The model under review builds one solid part; all positions refer to its coordinate system, in mm. A direction names the side the tool comes from. Round coordinates to 2 decimals unless told otherwise and drop trailing zeros. Order: outer loops, then holes, each group sorted by start corner. A loop starts at its lowest first (then second) coordinate and runs counter-clockwise, first axis right, second up. Notation, with made-up numbers: (64, -22.75) -> (70, -22.75) arc R12 cw to (70, -11.75) -> close; hole circle Ø5 at (32.5, 49). An arc over 180 degrees is marked (long way). Return JSON: item names as keys, results as strings. Group by question number.
from build123d import *

# Parameters (mm, degrees)
MODEL_R             = 1.6
MODEL_R_2           = 1.5
MODEL_W             = 10.2
MODEL_H             = 3.5
MODEL_W_2           = 4.5
MODEL_H_2           = 10.2
MODEL_W_3           = 3.5
BOSS_EXTRUDE1_DEPTH = 3


with BuildPart() as part:
    # Model → Boss-Extrude1 (new body)
    with BuildSketch(Plane.XY):
        with BuildLine():
            Line((6.5, -85.9), (88.4, -85.9))
            ThreePointArc((88.4, -85.9), (95.471067812, -82.971067812), (98.4, -75.9))
            Line((98.4, -75.9), (98.4, -6.5))
            ThreePointArc((98.4, -6.5), (95.471067812, 0.571067812), (88.4, 3.5))
            Line((88.4, 3.5), (6.5, 3.5))
            ThreePointArc((6.5, 3.5), (-0.571067812, 0.571067812), (-3.5, -6.5))
            Line((-3.5, -6.5), (-3.5, -75.9))
            ThreePointArc((-3.5, -75.9), (-0.571067812, -82.971067812), (6.5, -85.9))
        make_face()
        with Locations((35.64, -17.27)):
            Circle(MODEL_R, mode=Mode.SUBTRACT)
        with Locations((34.37, -65.53)):
            Circle(MODEL_R, mode=Mode.SUBTRACT)
        with Locations((22.5, -78.9)):
            Circle(MODEL_R_2, mode=Mode.SUBTRACT)
        with Locations((72.4, -3.5)):
            Circle(MODEL_R_2, mode=Mode.SUBTRACT)
        with Locations((22.5, -3.5)):
            Circle(MODEL_R_2, mode=Mode.SUBTRACT)
        with Locations((72.4, -78.9)):
            Circle(MODEL_R_2, mode=Mode.SUBTRACT)
        with Locations((86.44, -32.51)):
            Circle(MODEL_R, mode=Mode.SUBTRACT)
        with Locations((59.8, -79.15)):
            Rectangle(MODEL_W, MODEL_H, mode=Mode.SUBTRACT)
        with Locations((10.1, -79.15)):
            Rectangle(MODEL_W, MODEL_H, mode=Mode.SUBTRACT)
        with Locations((59.8, -3.25)):
            Rectangle(MODEL_W, MODEL_H, mode=Mode.SUBTRACT)
        with Locations((10.1, -3.25)):
            Rectangle(MODEL_W, MODEL_H, mode=Mode.SUBTRACT)
        with Locations((2.75, -41.2)):
            Rectangle(MODEL_W_2, MODEL_H_2, mode=Mode.SUBTRACT)
        with Locations((91.65, -41.2)):
            Rectangle(MODEL_W_3, MODEL_H_2, mode=Mode.SUBTRACT)
        with Locations((35.1, -3.25)):
            Rectangle(MODEL_W, MODEL_H, mode=Mode.SUBTRACT)
        with Locations((84.8, -3.25)):
            Rectangle(MODEL_W, MODEL_H, mode=Mode.SUBTRACT)
        with Locations((35.1, -79.15)):
            Rectangle(MODEL_W, MODEL_H, mode=Mode.SUBTRACT)
        with Locations((84.8, -79.15)):
            Rectangle(MODEL_W, MODEL_H, mode=Mode.SUBTRACT)
    extrude(amount=BOSS_EXTRUDE1_DEPTH)


solid = part.part
Item 1: Wall thickness on line 1 along Y through (x, z) = (84.5, 0.75); line 2 along X through (y, z) = (-42, 0.25); line 3 along Y through (x, z) = (22.5, 1.55): over which ranges is each line inside the solid? List them lowest first.
Item 2: For faces 4 (the face through (35, -77.4, 1)), 5 (the face through (47, -85.9, 1)), list the 3-axis set-ups (+Z, -Z, +X, -X, +Y, -Y) from which the entire face can be reached by the end or side of a thin tool; tool diameter is ignored.
Item 3: Consider section C-C on x = 86.44. State the section outline as (y, z) points, plus the area to 3 significant figures.
Item 4: Consider section A-A on x = 72.4. State the section outline as (y, z) points.
Item 5: Insertion check: pin 1 Ø0.9 at (y, z) = (-3, 2) entering from -X; pin 2 Ø0.9 at (x, z) = (92.5, 1) entering from +Y; pin 3 Ø0.9 at (y, z) = (-78.5, 2) entering from +X. Each pin has a flat end and moves straight along its axis. Give the tip position at first contact, or say it passes through.
Item 6: The part is to be moulded in two halves that separate along Y. For faces 1 (the face through (85, -77.4, 1)), 2 (the face through (93.4, -41, 1)), 3 (the face through (-0.65, -82.89, 1.48)), say which applies: +Y half, -Y half, draft (parallel to the pull), parting line (faces both ways), or undercut.
Item 7: Consider section B-B on y = -65.53. State the section outline as (x, z) points.
Item 8: Consider section D-D on y = -3.5. State the section outline as (x, z) points, plus the area to 3 significant figures.
Values:
{
 "1": {"line 1": "-85.9 to -80.9, -77.4 to -5, -1.5 to 3.5", "line 2": "-3.5 to 0.5, 5 to 89.9, 93.4 to 98.4", "line 3": "-85.9 to -80.4, -77.4 to -5, -2 to 3.5"},
 "2": {"face 4": "+Z, -Z", "face 5": "+Z, -Z, +X, -X, -Y"},
 "3": {"outline": "(-85.9, 0) -> (-80.9, 0) -> (-80.9, 3) -> (-85.9, 3) -> close; (-77.4, 0) -> (-34.11, 0) -> (-34.11, 3) -> (-77.4, 3) -> close; (-30.91, 0) -> (-5, 0) -> (-5, 3) -> (-30.91, 3) -> close; (-1.5, 0) -> (3.5, 0) -> (3.5, 3) -> (-1.5, 3) -> close", "area": "238 mm^2"},
 "4": {"outline": "(-85.9, 0) -> (-80.4, 0) -> (-80.4, 3) -> (-85.9, 3) -> close; (-77.4, 0) -> (-5, 0) -> (-5, 3) -> (-77.4, 3) -> close; (-2, 0) -> (3.5, 0) -> (3.5, 3) -> (-2, 3) -> close"},
 "5": {"pin 1": "x = -3.02", "pin 2": "y = 2.81", "pin 3": "x = 98.17"},
 "6": {"face 1": "undercut", "face 2": "undercut", "face 3": "-Y half"},
 "7": {"outline": "(-3.5, 0) -> (32.77, 0) -> (32.77, 3) -> (-3.5, 3) -> close; (35.97, 0) -> (98.4, 0) -> (98.4, 3) -> (35.97, 3) -> close"},
 "8": {"outline": "(-3.04, 0) -> (5, 0) -> (5, 3) -> (-3.04, 3) -> close; (15.2, 0) -> (21, 0) -> (21, 3) -> (15.2, 3) -> close; (24, 0) -> (30, 0) -> (30, 3) -> (24, 3) -> close; (40.2, 0) -> (54.7, 0) -> (54.7, 3) -> (40.2, 3) -> close; (64.9, 0) -> (70.9, 0) -> (70.9, 3) -> (64.9, 3) -> close; (73.9, 0) -> (79.7, 0) -> (79.7, 3) -> (73.9, 3) -> close; (89.9, 0) -> (97.94, 0) -> (97.94, 3) -> (89.9, 3) -> close", "area": "163 mm^2"}
}
